Check sheet for the modelled part. Datum: model origin and axes. Units: mm. A direction names the side the tool comes from. Round coordinates to 2 decimals unless told otherwise and drop trailing zeros. Loops run counter-clockwise (first coordinate to the right, second up) from the corner with the lowest first, then second, coordinate; pieces in that order, holes last. Notation, with made-up numbers: (71, 55) - (78, 55) arc R8 cw to (78, 63) - close; hole circle Ø9 at (-39, -34.5). An arc over 180 degrees is marked (long way). Put each result on its own line as item: value. Start each with the question number.
Item 1: Material ranges on line 1 along X through (y, z) = (38, 25); line 2 along X through (y, z) = (32, -4.5); line 3 along Y through (x, z) = (16.5, -13), recorded low to high.
Item 2: Tool access check on faces 1 (the cylindrical face through (17.46, 99.66, 5.21)), 2 (the cylindrical face through (55, 25.12, 1.08)), 3 (the cylindrical face through (5.14, 67.436, 0.976)). Record the directions out of +Z, -Z, +X, -X, +Y, -Y that give a thin tool (end or side, any length) a straight path to the whole face; none if there is none.
Item 3: Section check D-D, the plane y = 33.5. Record the cut outline in (x, z).
Item 4: Section check C-C, the plane x = 4.5. Record the cut outline in (y, z), and give its area (3 significant figures).
Item 5: Section check A-A, the plane y = 60. Record the cut outline in (x, z), and give its area (3 significant figures).
Item 6: Gauge pin test, flat ends, axial feed: pin 1 Ø3 at (x, y) = (27, 34.5) entering from -Z; pin 2 Ø10 at (y, z) = (53, -22.5) entering from +X; pin 3 Ø10 at (x, y) = (14, 71) entering from -Z. Record the tip position at first contact, or that the pin passes through.
Item 7: Section check B-B, the plane z = 0. Record the cut outline in (x, y), and give its area (3 significant figures).
from build123d import *

# Parameters (mm, degrees)
SKETCH2_R                = 7.5
BOSS_EXTRUDE1_DEPTH      = 5
BOSS_EXTRUDE1_DEPTH_BACK = 15
SKETCH3_R                = 40
BOSS_EXTRUDE2_DEPTH      = 5
SKETCH4_R                = 5
BOSS_EXTRUDE3_DEPTH      = 70.98805519


with BuildPart() as part:
    # Sketch2 → Boss-Extrude1 (new body, two sides)
    with BuildSketch(Plane(origin=(10, 0, 0), x_dir=(0, 0, -1), z_dir=(1, 0, 0))) as boss_extrude1_sk:
        with Locations((0, 60)):
            Circle(SKETCH2_R)
    extrude(amount=BOSS_EXTRUDE1_DEPTH)
    extrude(boss_extrude1_sk.sketch, amount=-BOSS_EXTRUDE1_DEPTH_BACK)

    # Sketch3 → Boss-Extrude2 (add)
    with BuildSketch(Plane(origin=(15, 0, 0), x_dir=(0, 0, -1), z_dir=(1, 0, 0))):
        with Locations((0, 60)):
            Circle(SKETCH3_R)
    extrude(amount=BOSS_EXTRUDE2_DEPTH)

    # Sketch4 → Boss-Extrude3 (add)
    with BuildSketch(Plane(origin=(20, 0, 0), x_dir=(0, 0, -1), z_dir=(1, 0, 0))):
        with Locations((0, 30)):
            Circle(SKETCH4_R)
    extrude(amount=BOSS_EXTRUDE3_DEPTH)


solid = part.part
Check result:
1. line 1: 15 to 20
1. line 2: 15 to 90.99
1. line 3: 22.17 to 97.83
2. face 1: +X, -X
2. face 2: +X
2. face 3: -X
3. outline: (15, -29.96) - (20, -29.96) - (20, -3.57) - (90.99, -3.57) - (90.99, 3.57) - (20, 3.57) - (20, 29.96) - (15, 29.96) - close
4. outline: circle Ø15 at (60, 0)
4. area: 177 mm²
5. outline: (-5, -7.5) - (15, -7.5) - (15, -40) - (20, -40) - (20, 40) - (15, 40) - (15, 7.5) - (-5, 7.5) - close
5. area: 700 mm²
6. pin 1: z = -4
6. pin 2: x = 20
6. pin 3: z = -39.53
7. outline: (-5, 52.5) - (15, 52.5) - (15, 20) - (20, 20) - (20, 25) - (90.99, 25) - (90.99, 35) - (20, 35) - (20, 100) - (15, 100) - (15, 67.5) - (-5, 67.5) - close
7. area: 1,410 mm²
